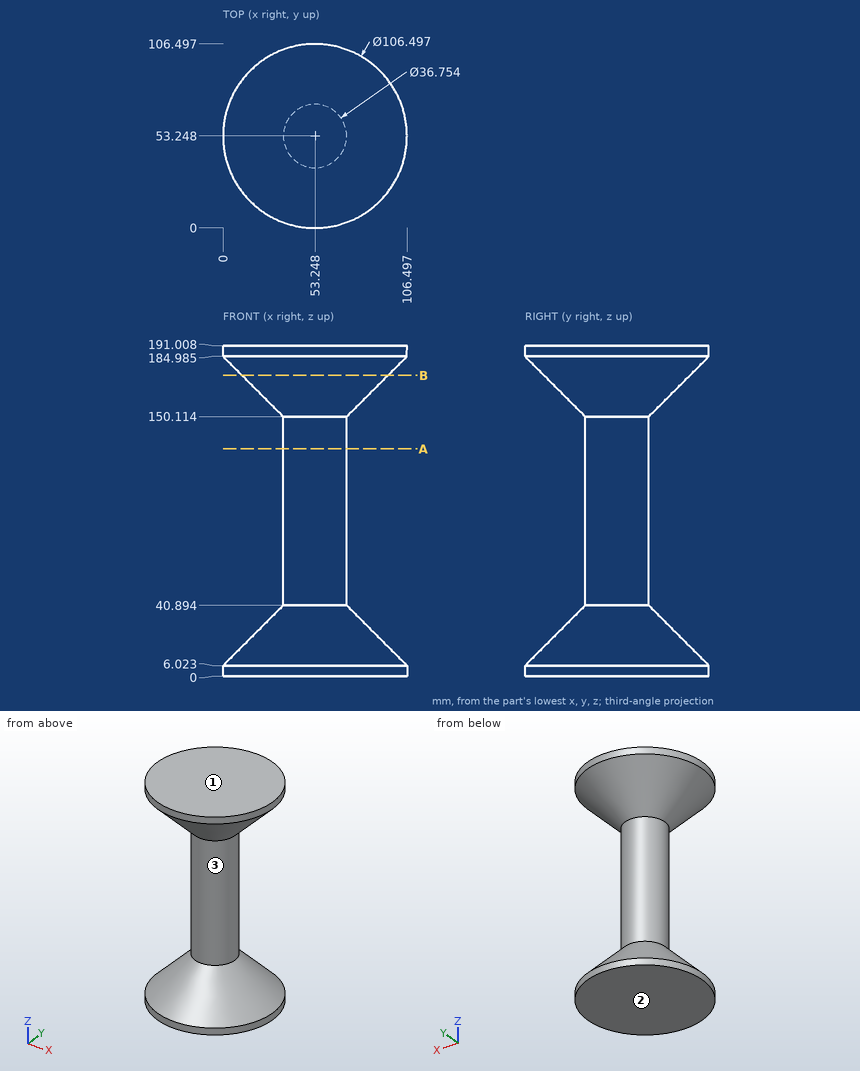
Design review of the part shown in the three views and the two pictorial views. Dimensions are in mm from the part's minimum x, y and z. Coordinates: 2 decimals unless noted, no trailing zeros. Order: outer loops, then holes, each group sorted by start corner. A loop starts at its lowest first (then second) coordinate and runs counter-clockwise, first axis right, second up.
1) Mouldability with a two-part tool opening along Z and no side actions: class the marked faces 1, 2 and 3 as +Z half, -Z half, draft (parallel to the pull), parting line (faces both ways), or undercut.
2) Clearance check with flat-ended pins moving along their axes: pin 1 (8 mm diameter, centred on y = 76, z = 126.5, fed in from -X); pin 2 (5 mm diameter, centred on x = 47.5, y = 48.5, fed in from -Z); pin 3 (5 mm diameter, centred on y = 43.5, z = 27.5, fed in from -X) (1 decimal); pin 4 (12 mm diameter, centred on x = 52.5, z = 73.5, fed in from +Y) (1 decimal). State where each tip first meets the part, or that it passes through.
3) Wall thickness on line 1 along Z through (x, y) = (50.5, 72.5) (1 decimal); line 2 along Z through (x, y) = (90.5, 28); line 3 along Y through (x, z) = (53, 58.5): over which ranges is each line inside the solid? List them lowest first.
4) Take a section at A-A, the plane z = 131.5. Give the boundary of the cut face in (x, y) (1 decimal), and give its area (3 significant figures).
5) Take a section at B-B, the plane z = 174. Give the boundary of the cut face in (x, y), and give its area (3 significant figures).
Returned:
1. face 1: +Z half
1. face 2: -Z half
1. face 3: undercut
2. pin 1: passes through
2. pin 2: stops at z = 0
2. pin 3: stops at x = 20.3
2. pin 4: stops at y = 71.6
3. line 1: z = 0 to 39.8, 151.2 to 191
3. line 2: z = 0 to 14.27, 176.74 to 191.01
3. line 3: y = 34.87 to 71.62
4. outline: circle Ø36.8 at (53.2, 53.2)
4. area: 1,060 mm2
5. outline: circle Ø84.53 at (53.25, 53.25)
5. area: 5,610 mm2
